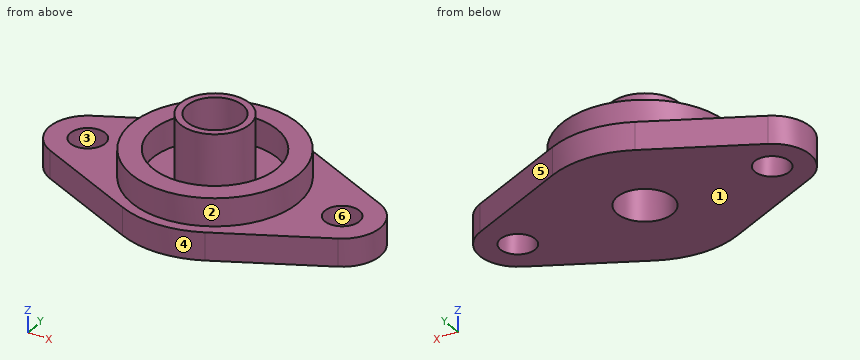
```python
from build123d import *

# Parameters (mm, degrees)
SKETCH_R      = 2.5
PAD_DEPTH     = 4
SKETCH001_R   = 5
PAD001_DEPTH  = 9
SKETCH002_R   = 4
POCKET_DEPTH  = 13.001
SKETCH003_R   = 12
SKETCH003_R_2 = 9
PAD002_DEPTH  = 4


with BuildPart() as part:
    # Sketch → Pad (new body)
    with BuildSketch(Plane.XY):
        with BuildLine():
            ThreePointArc((-20.660959, 4.943407), (-23.75, 0), (-20.660959, -4.943407))
            Line((-5.917808, -12.133818), (-20.660959, -4.943407))
            ThreePointArc((-5.917808, -12.133818), (0, -13.5), (5.917808, -12.133818))
            Line((20.660959, -4.943407), (5.917808, -12.133818))
            ThreePointArc((20.660959, -4.943407), (23.75, 0), (20.660959, 4.943407))
            Line((5.917808, 12.133818), (20.660959, 4.943407))
            ThreePointArc((5.917808, 12.133818), (0, 13.5), (-5.917808, 12.133818))
            Line((-20.660959, 4.943407), (-5.917808, 12.133818))
        make_face()
        with Locations((-18.25, 0)):
            Circle(SKETCH_R, mode=Mode.SUBTRACT)
        with Locations((18.25, 0)):
            Circle(SKETCH_R, mode=Mode.SUBTRACT)
    extrude(amount=PAD_DEPTH)

    # Sketch001 (on Face12 of Pad) → Pad001 (join)
    with BuildSketch(Plane.XY.offset(4)):
        Circle(SKETCH001_R)
    extrude(amount=PAD001_DEPTH)

    # Sketch002 (on Face14 of Pad001) → Pocket (cut, through all)
    with BuildSketch(Plane.XY.offset(13)):
        Circle(SKETCH002_R)
    extrude(amount=-POCKET_DEPTH, mode=Mode.SUBTRACT)

    # Sketch003 (on Face5 of Pocket) → Pad002 (join)
    with BuildSketch(Plane.XY.offset(4)):
        Circle(SKETCH003_R)
        Circle(SKETCH003_R_2, mode=Mode.SUBTRACT)
    extrude(amount=PAD002_DEPTH)


solid = part.part
```
Source: CAD feature listing. Evaluate the final solid. Frame: model axes, mm. Face numbers are marked on the shaded views. A direction names the side the tool comes from. Give positions to 0.01 mm unless a question says otherwise; leave off trailing zeros. Loops run counter-clockwise (first coordinate to the right, second up) from the corner with the lowest first, then second, coordinate; pieces in that order, holes last. Notation, with made-up numbers: (70.25, 44) -> (120.25, 44) arc R19 cw to (120.25, 59) -> close; hole circle Ø7 at (20, -9.5). An arc over 180 degrees is marked (long way). Put each result on its own line as item: value. Start each with the question number.
1) Draft query along X for the marked faces 3, 4, 5 and 6. Return one class per face: released by +X, released by -X, zero draft, split by the parting line, or undercut.
2) Material intervals for probe 1 along Y at (x, z) = (0, 4.25); probe 2 along X at (y, z) = (-2.75, 6); probe 3 along X at (y, z) = (-0.5, 0.75), sorted ascending.
3) Reachability of the marked faces 1 and 2 from +Z, -Z, +X, -X, +Y, -Y: full face, straight path, thin tool, end or side. Return the list, or none.
4) Contact query for flat-ended pins moving along their axis: P1, Ø14.5, axis at x = 0.5, y = 1, coming from the +Z side; P2, Ø10, axis at x = -10, y = 2, coming from the +Z side; P3, Ø8, axis at x = 18.25, y = 0, coming from the +Z side. Output: stop coordinate, or through.
5) Cut plane A-A (y = 0). Return loops of the section in (x, z), then the cut area to 3 significant figures.
6) Cut plane D-D (z = 10). Return loops of the section in (x, y).
7) Cut plane B-B (x = 0). Return loops of the section in (y, z), then the cut area to 3 significant figures.
8) Cut plane C-C (z = 3.5). Return loops of the section in (x, y), then the cut area to 3 significant figures.
Results are:
1. face 3: undercut
1. face 4: split by the parting line
1. face 5: released by +X
1. face 6: undercut
2. probe 1: y = -12 to -9, -5 to -4, 4 to 5, 9 to 12
2. probe 2: x = -11.68 to -8.57, -4.18 to -2.9, 2.9 to 4.18, 8.57 to 11.68
2. probe 3: x = -23.73 to -20.7, -15.8 to -3.97, 3.97 to 15.8, 20.7 to 23.73
3. face 1: -Z, +X, -X, +Y, -Y
3. face 2: +Z
4. P1: stops at z = 13
4. P2: stops at z = 8
4. P3: stops at z = 4
5. outline: (-23.75, 0) -> (-20.75, 0) -> (-20.75, 4) -> (-23.75, 4) -> close; (-15.75, 0) -> (-4, 0) -> (-4, 13) -> (-5, 13) -> (-5, 4) -> (-9, 4) -> (-9, 8) -> (-12, 8) -> (-12, 4) -> (-15.75, 4) -> close; (4, 0) -> (15.75, 0) -> (15.75, 4) -> (12, 4) -> (12, 8) -> (9, 8) -> (9, 4) -> (5, 4) -> (5, 13) -> (4, 13) -> close; (20.75, 0) -> (23.75, 0) -> (23.75, 4) -> (20.75, 4) -> close
5. area: 160 mm2
6. outline: circle Ø10 at (0, 0); hole circle Ø8 at (0, 0)
7. outline: (-13.5, 0) -> (-4, 0) -> (-4, 13) -> (-5, 13) -> (-5, 4) -> (-9, 4) -> (-9, 8) -> (-12, 8) -> (-12, 4) -> (-13.5, 4) -> close; (4, 0) -> (13.5, 0) -> (13.5, 4) -> (12, 4) -> (12, 8) -> (9, 8) -> (9, 4) -> (5, 4) -> (5, 13) -> (4, 13) -> close
7. area: 118 mm2
8. outline: (-20.66, -4.94) -> (-5.92, -12.13) arc R13.5 ccw to (5.92, -12.13) -> (20.66, -4.94) arc R5.5 ccw to (20.66, 4.94) -> (5.92, 12.13) arc R13.5 ccw to (-5.92, 12.13) -> (-20.66, 4.94) arc R5.5 ccw to start; hole circle Ø5 at (-18.25, 0); hole circle Ø8 at (0, 0); hole circle Ø5 at (18.25, 0)
8. area: 767 mm2
